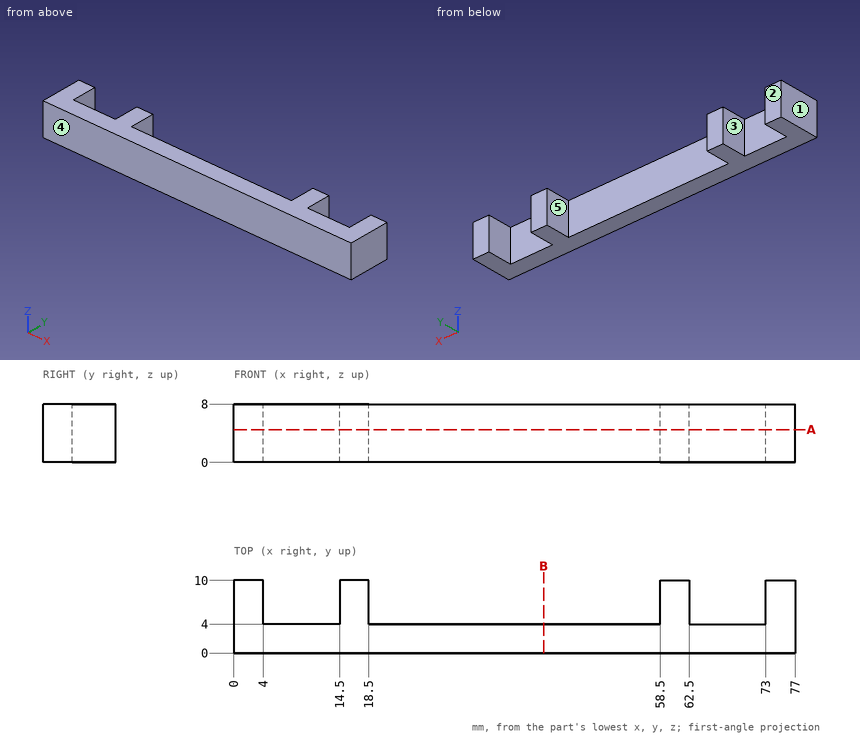
Verification items for this drawing (mm, ordinates from the low corner). A direction names the side the tool comes from. Round coordinates to 2 decimals unless told otherwise and drop trailing zeros. Order: outer loops, then holes, each group sorted by start corner. A loop starts at its lowest first (then second) coordinate and runs counter-clockwise, first axis right, second up. Notation, with made-up numbers: (14, 5) - (73, 5) arc R8 ccw to (73, 13) - close; hole circle Ø6 at (-17, 38). An arc over 180 degrees is marked (long way). Use CSV: the item, a comma, the result in double quotes.
(1) Thickness scan on probe 1 along X at (y, z) = (9.25, 7.5); probe 2 along Y at (x, z) = (35, 5). Record the ranges inside material, lowest first. Write a range as from..to.
Entries:
probe 1,"0..4, 14.5..18.5, 58.5..62.5, 73..77"
probe 2,"0..4"
(2) Access from +Z, -Z, +X, -X, +Y, -Y to the whole of each face (thin tool, end or side, straight path). Record for the marked faces 4 and 5.
Entries:
face 4,"+Z, -Z, +X, -X, -Y"
face 5,"+Z, -Z, +Y"
(3) Section check A-A on z = 4.5. Record the boundary of the cut face in (x, y).
Entries:
outline,"(0, 0) - (77, 0) - (77, 10) - (73, 10) - (73, 4) - (62.5, 4) - (62.5, 10) - (58.5, 10) - (58.5, 4) - (18.5, 4) - (18.5, 10) - (14.5, 10) - (14.5, 4) - (4, 4) - (4, 10) - (0, 10) - close"
(4) Gauge pin test, flat ends, axial feed: pin 1 Ø4 at (x, z) = (42.5, 2.5) entering from +Y; pin 2 Ø5 at (x, y) = (67, 5) entering from -Z. Record the tip position at first contact, or that the pin passes through.
Entries:
pin 1,"y = 4"
pin 2,"z = 0"
(5) Mould release check, pull along X, two halves, no side actions. Record for the marked faces 1, 2 and 3: released by +X, released by -X, zero draft, split by the parting line, or undercut.
Entries:
face 1,"released by -X"
face 2,"zero draft"
face 3,"undercut"
(6) Section check B-B on x = 42.5. Record the boundary of the cut face in (y, z), and give its area (3 significant figures).
Entries:
outline,"(0, 0) - (4, 0) - (4, 8) - (0, 8) - close"
area,"32.0 mm^2"
